Verification items for the finished model (mm, model axes). A direction names the side the tool comes from. Round coordinates to 2 decimals unless told otherwise and drop trailing zeros. Order: outer loops, then holes, each group sorted by start corner. A loop starts at its lowest first (then second) coordinate and runs counter-clockwise, first axis right, second up. Notation, with made-up numbers: M 52.25,45.5 L 109.25,45.5 A9 ccw 109.25,60.5 Z; hole C 65,0.25 d11. An arc over 180 degrees is marked long. Use CSV: the item, a comma, the result in double quotes. Start each with the question number.
Q1. Set-up check for faces 1 (the face through (-52.91, 30.37, 1.48)), 2 (the face through (102.285, -22.589, 1.479)), 3 (the face through (91.28, -39.75, 1.48)), 4 (the face through (-105.027, 0.896, 1.479)), 5 (the face through (91.946, 41.034, 1.479)): record each of +Z, -Z, +X, -X, +Y, -Y from which the full face is reachable in a straight line by a thin tool's end or side.
Q2. Mould release check, pull along X, two halves, no side actions. Record for faces 6 (the face through (-1, 11, 3)), 7 (the face through (53.52, 30.89, 1.48)), 8 (the face through (0.648, 106.014, 1.479)): +X half, -X half, draft (parallel to the pull), parting line (faces both ways), or undercut.
Q3. Sectioned sample at C-C (x = 42). Enter the section's corners in (y, z), and give its area (3 significant figures).
Q4. Scan lines: line 1 (X direction, y = 7.5, z = 0.35); line 2 (Y direction, x = -46.5, z = 1.9); line 3 (X direction, y = -44.5, z = 0.6). Record each from-to range of solid material in increasing order.
Q5. Sectioned sample at D-D (z = 1). State how many separate pieces and enclosed holes the cut face has, and give its area (3 significant figures).
Q6. Sectioned sample at A-A (y = -11.5). Enter the section's corners in (x, z).
Q7. Sectioned sample at B-B (y = 67). Enter the section's corners in (x, z), and give its area (3 significant figures).
Q8. Gauge pin test, flat ends, axial feed: pin 1 Ø0.9 at (x, z) = (-77, 2) entering from -Y; pin 2 Ø15 at (x, y) = (-91.34, -22.45) entering from -Z; pin 3 Ø0.9 at (x, z) = (0.5, 1) entering from -Y; pin 4 Ø1 at (y, z) = (-11, 2.5) entering from +X. Record the tip position at first contact, or that the pin passes through.
```python
from build123d import *

# Parameters (mm, degrees)
F0_R     = 6.5
F1_DEPTH = 3


with BuildPart() as f1:
    # F0 (on Top) → F1 (new body)
    with BuildSketch(Plane.XY):
        with BuildLine():
            ThreePointArc((104.967828, 0), (104.971515, 0.508028), (104.972745, 1.016069))
            ThreePointArc((104.972745, 1.016069), (102.578155, 23.312476), (95.503606, 44.591917))
            Line((95.503606, 44.591917), (88.286917, 37.375229))
            Line((88.286917, 37.375229), (74.144781, 51.517364))
            Line((74.144781, 51.517364), (32.312379, 9.684962))
            Line((32.312379, 9.684962), (20.998671, 20.998671))
            Line((20.998671, 20.998671), (9.684962, 32.312379))
            Line((9.684962, 32.312379), (51.67823, 74.305647))
            Line((51.67823, 74.305647), (37.536094, 88.447782))
            Line((37.536094, 88.447782), (44.972721, 95.88441))
            ThreePointArc((44.972721, 95.88441), (-0.002561, 106.016066), (-44.982604, 95.905566))
            Line((-44.982604, 95.905566), (-37.562306, 88.504525))
            Line((-37.562306, 88.504525), (-51.686055, 74.344027))
            Line((-51.686055, 74.344027), (-9.657337, 32.424378))
            Line((-9.657337, 32.424378), (-20.956336, 21.09598))
            Line((-20.956336, 21.09598), (-32.255336, 9.767582))
            Line((-32.255336, 9.767582), (-74.161182, 51.564677))
            Line((-74.161182, 51.564677), (-88.284931, 37.404179))
            Line((-88.284931, 37.404179), (-95.537237, 44.637663))
            ThreePointArc((-95.537237, 44.637663), (-105.024504, 0.255865), (-94.895596, -43.983908))
            Line((-94.895596, -43.983908), (-87.458969, -36.547281))
            Line((-87.458969, -36.547281), (-73.316833, -50.689416))
            Line((-73.316833, -50.689416), (-31.323566, -8.696149))
            Line((-31.323566, -8.696149), (-20.009857, -20.009857))
            Line((-20.009857, -20.009857), (-8.696149, -31.323566))
            Line((-8.696149, -31.323566), (-50.528551, -73.155968))
            Line((-50.528551, -73.155968), (-37.529173, -86.155346))
            Line((-37.529173, -86.155346), (-26.15007, -74.776243))
            Line((-26.15007, -74.776243), (0, -74.776243))
            Line((0, -74.776243), (26.095559, -74.776243))
            Line((26.095559, -74.776243), (37.596906, -86.277589))
            Line((37.596906, -86.277589), (50.853229, -72.895181))
            Line((50.853229, -72.895181), (8.819452, -31.257433))
            Line((8.819452, -31.257433), (20.079485, -19.890303))
            Line((20.079485, -19.890303), (31.339518, -8.523172))
            Line((31.339518, -8.523172), (73.527238, -50.313413))
            Line((73.527238, -50.313413), (87.60228, -36.1045))
            Line((87.60228, -36.1045), (95.068799, -43.500673))
            ThreePointArc((95.068799, -43.500673), (102.355326, -22.282148), (104.967828, 0))
        make_face()
        with Locations((-91.341169, -22.449345)):
            Circle(F0_R, mode=Mode.SUBTRACT)
        with Locations((91.286659, -22.449345)):
            Circle(F0_R, mode=Mode.SUBTRACT)
        with BuildLine():
            Line((-68.135568, 0), (-82.135568, 0))
            ThreePointArc((-82.135568, 0), (-84.256888, 0.87868), (-85.135568, 3))
            Line((-85.135568, 3), (-85.135568, 17))
            ThreePointArc((-85.135568, 17), (-84.256888, 19.12132), (-82.135568, 20))
            Line((-82.135568, 20), (-68.135568, 20))
            ThreePointArc((-68.135568, 20), (-66.014247, 19.12132), (-65.135568, 17))
            Line((-65.135568, 17), (-65.135568, 3))
            ThreePointArc((-65.135568, 3), (-66.014247, 0.87868), (-68.135568, 0))
        make_face(mode=Mode.SUBTRACT)
        with Locations((-29.749685, 90.793084)):
            Circle(F0_R, mode=Mode.SUBTRACT)
        with BuildLine():
            ThreePointArc((85.104936, 3), (84.226257, 0.87868), (82.104936, 0))
            Line((82.104936, 0), (68.104936, 0))
            ThreePointArc((68.104936, 0), (65.983616, 0.87868), (65.104936, 3))
            Line((65.104936, 3), (65.104936, 17))
            ThreePointArc((65.104936, 17), (65.983616, 19.12132), (68.104936, 20))
            Line((68.104936, 20), (82.104936, 20))
            ThreePointArc((82.104936, 20), (84.226257, 19.12132), (85.104936, 17))
            Line((85.104936, 17), (85.104936, 3))
        make_face(mode=Mode.SUBTRACT)
        with BuildLine():
            Line((7, 54.305647), (0, 54.305647))
            Line((0, 54.305647), (-7, 54.305647))
            ThreePointArc((-7, 54.305647), (-9.12132, 55.184326), (-10, 57.305647))
            Line((-10, 57.305647), (-10, 71.305647))
            ThreePointArc((-10, 71.305647), (-9.12132, 73.426967), (-7, 74.305647))
            Line((-7, 74.305647), (0, 74.305647))
            Line((0, 74.305647), (7, 74.305647))
            ThreePointArc((7, 74.305647), (9.12132, 73.426967), (10, 71.305647))
            Line((10, 71.305647), (10, 57.305647))
            ThreePointArc((10, 57.305647), (9.12132, 55.184326), (7, 54.305647))
        make_face(mode=Mode.SUBTRACT)
        with Locations((29.269962, 90.793084)):
            Circle(F0_R, mode=Mode.SUBTRACT)
    extrude(amount=F1_DEPTH)


solid = f1.part
```
Verdict:
1,face 1,"+Z, -Z"
1,face 2,"+Z, -Z, +X, -Y"
1,face 3,"+Z, -Z, -Y"
1,face 4,"+Z, -Z, -X"
1,face 5,"+Z, -Z, +Y"
2,face 6,"draft"
2,face 7,"undercut"
2,face 8,"parting line"
3,outline,"M -81.83,0 L -64.13,0 L -64.13,3 L -81.83,3 Z; M -19.08,0 L 19.37,0 L 19.37,3 L -19.08,3 Z; M 64.63,0 L 83.98,0 L 83.98,3 L 64.63,3 Z; M 92.91,0 L 97.24,0 L 97.24,3 L 92.91,3 Z"
3,area,"240 mm²"
4,line 1,"x = -104.83 to -85.14, -65.14 to 65.1, 85.1 to 104.77"
4,line 2,"y = -77.18 to -69.13, -23.87 to 23.98, 69.17 to 79.54"
4,line 3,"x = -79.51 to -67.13, -21.87 to 22.19, 67.66 to 79.29"
5,separate pieces,"1"
5,enclosed holes,"7"
5,area,"19,200 mm²"
6,outline,"M -104.28,0 L -34.13,0 L -34.13,3 L -104.28,3 Z; M -28.52,0 L 28.39,0 L 28.39,3 L -28.52,3 Z; M 34.34,0 L 104.22,0 L 104.22,3 L 34.34,3 Z"
7,outline,"M -44.32,0 L -10,0 L -10,3 L -44.32,3 Z; M 10,0 L 44.37,0 L 44.37,3 L 10,3 Z"
7,area,"206 mm²"
8,pin 1,"stops at y = -47.46"
8,pin 2,"stops at z = 0"
8,pin 3,"stops at y = -74.78"
8,pin 4,"stops at x = 104.34"
